from build123d import *

# Parameters (mm, degrees)
SKETCH1_R           = 1.5
SKETCH1_R_2         = 2.25
BOSS_EXTRUDE1_DEPTH = 8
CHAMFER1_SIZE       = 1.75
CUT_EXTRUDE1_DEPTH  = 2
SKETCH4_R           = 3
CUT_EXTRUDE2_DEPTH  = 3
FILLET1_R           = 0.7
FILLET2_R           = 0.5


with BuildPart() as part:
    # Sketch1 → Boss-Extrude1 (new body)
    with BuildSketch(Plane(origin=(0, 0, 0), x_dir=(1, 0, 0), z_dir=(0, 1, 0))):
        with BuildLine():
            Line((-22.5, 10), (22.5, 10))
            ThreePointArc((22.5, 10), (32.5, 0), (22.5, -10))
            Line((22.5, -10), (-22.5, -10))
            ThreePointArc((-22.5, -10), (-32.5, 0), (-22.5, 10))
        make_face()
        with Locations(Location((-22.5, 0, 0), (0, 0, 270))):
            Circle(SKETCH1_R, mode=Mode.SUBTRACT)
        with Locations(Location((22.5, 0, 0), (0, 0, 270))):
            Circle(SKETCH1_R, mode=Mode.SUBTRACT)
        with Locations(Location((0, 0, 0), (0, 0, 270))):
            Circle(SKETCH1_R_2, mode=Mode.SUBTRACT)
    extrude(amount=BOSS_EXTRUDE1_DEPTH)

    # Chamfer1
    chamfer1_edges = [part.edges().sort_by_distance(p)[0] for p in [
        (0, 8, -2.25),
    ]]
    chamfer(chamfer1_edges, length=CHAMFER1_SIZE)

    # Sketch3 → Cut-Extrude1 (cut)
    with BuildSketch(Plane.XZ):
        with BuildLine():
            Line((-10, 10), (-22.5, 10))
            ThreePointArc((-22.5, 10), (-32.5, 0), (-22.5, -10))
            Line((-22.5, -10), (-10, -10))
            Line((-10, -10), (-10, 10))
        make_face()
        with BuildLine():
            Line((22.5, 10), (10, 10))
            Line((10, 10), (10, -10))
            Line((10, -10), (22.5, -10))
            ThreePointArc((22.5, -10), (32.5, 0), (22.5, 10))
        make_face()
    extrude(amount=-CUT_EXTRUDE1_DEPTH, mode=Mode.SUBTRACT)

    # Sketch4 → Cut-Extrude2 (cut)
    with BuildSketch(Plane.XZ.offset(-2)):
        with Locations(Location((-22.5, 0, 0), (0, 0, 270))):
            Circle(SKETCH4_R)
        with Locations(Location((22.5, 0, 0), (0, 0, 270))):
            Circle(SKETCH4_R)
    extrude(amount=-CUT_EXTRUDE2_DEPTH, mode=Mode.SUBTRACT)

    # Fillet1
    fillet1_edges = [part.edges().sort_by_distance(p)[0] for p in [
        (-10, 0, 0),
        (-10, 2, 0),
        (10, 0, 0),
        (10, 2, 0),
    ]]
    fillet(fillet1_edges, radius=FILLET1_R)

    # Fillet2
    fillet2_edges = [part.edges().sort_by_distance(p)[0] for p in [
        (-22.5, 2, 3),
        (22.5, 2, 3),
    ]]
    fillet(fillet2_edges, radius=FILLET2_R)


solid = part.part
Verification items for the finished model (mm, model axes). A direction names the side the tool comes from. Round coordinates to 2 decimals unless told otherwise and drop trailing zeros. Loops run counter-clockwise (first coordinate to the right, second up) from the corner with the lowest first, then second, coordinate; pieces in that order, holes last. Notation, with made-up numbers: M -27,-2.75 L 18,-2.75 A23 cw 18,33.25 Z; hole C 62,7 d7. An arc over 180 degrees is marked long. Write each question's results on one line, items separated by ' | '.
1) Section check A-A on y = 3.25. Record the boundary of the cut face in (x, z).
Checks:
outline: M -22.5,-10 L 22.5,-10 A10 ccw 22.5,10 L -22.5,10 A10 ccw Z; hole C -22.5,0 d6; hole C 0,0 d4.5; hole C 22.5,0 d6
2) Mould release check, pull along Z, two halves, no side actions. Record for faces 4 (the cylindrical face through (32.5, 5, -0.2)), 5 (the flat face through (-19, 2, -2)), 6 (the flat face through (-21, 5, -1)): released by +Z, released by -Z, zero draft, split by the parting line, or undercut.
Checks:
face 4: split by the parting line | face 5: zero draft | face 6: undercut
3) Scan lines: L1, parallel to X at y = 3.6, z = 0; L2, parallel to X at y = 6.1, z = 0; L3, parallel to Z at x = 22.5, y = 6.1. Record each from-to range of solid material in increasing order. Write a range as from..to.
Checks:
L1: x = -32.5..-25.5, -19.5..-2.25, 2.25..19.5, 25.5..32.5 | L2: x = -32.5..-24, -21..-2.25, 2.25..21, 24..32.5 | L3: z = -10..-1.5, 1.5..10
4) Access from +Z, -Z, +X, -X, +Y, -Y to the whole of each face (thin tool, end or side, straight path). Record for faces 1 (the flat face through (19, 2, -2)), 2 (the cylindrical face through (-25.43, 3.73, 0.65)), 3 (the flat face through (0, 4, 10)).
Checks:
face 1: +Z, -Z, +X, -Y | face 2: -Y | face 3: +Z, +X, -X, +Y, -Y
5) Section check B-B on x = 13.5. Record the boundary of the cut face in (y, z).
Checks:
outline: M 2,-10 L 8,-10 L 8,10 L 2,10 Z
6) Section check C-C on z = 0. State how many separate pieces and enclosed holes the cut face has, then the cut area to 3 significant figures.
Checks:
separate pieces: 4 | enclosed holes: 0 | area: 337 mm2
7) Section check D-D on y = 7.25. Record the boundary of the cut face in (x, z), then the cut area to 3 significant figures.
Checks:
outline: M -22.5,-10 L 22.5,-10 A10 ccw 22.5,10 L -22.5,10 A10 ccw Z; hole C -22.5,0 d3; hole C 0,0 d6.5; hole C 22.5,0 d3 | area: 1,170 mm2
8) Gauge pin test, flat ends, axial feed: P1, Ø3.5, axis at x = 22.5, z = 0, coming from the +Y side; P2, Ø3.5, axis at x = 0, z = 0, coming from the +Y side; P3, Ø8, axis at x = 22.5, z = 0, coming from the -Y side; P4, Ø3, axis at y = 1, z = -3.5, coming from the -X side. Record the tip position at first contact, or that the pin passes through.
Checks:
P1: stops at y = 8 | P2: passes through | P3: stops at y = 2 | P4: stops at x = -32.21
